```python
from build123d import *

# Parameters (mm, degrees)
SKETCH1_R           = 2.5
BOSS_EXTRUDE1_DEPTH = 45
SKETCH2_R           = 2.5
SKETCH2_R_2         = 2
CUT_EXTRUDE1_DEPTH  = 8
SKETCH3_R           = 2.5
SKETCH3_R_2         = 2
CUT_EXTRUDE2_DEPTH  = 8


with BuildPart() as part:
    # Sketch1 → Boss-Extrude1 (new body, symmetric)
    with BuildSketch(Plane(origin=(0, 0, 0), x_dir=(0, 0, -1), z_dir=(1, 0, 0))):
        Circle(SKETCH1_R)
    extrude(amount=BOSS_EXTRUDE1_DEPTH, both=True)

    # Sketch2 → Cut-Extrude1 (cut)
    with BuildSketch(Plane(origin=(45, 0, 0), x_dir=(0, 0, -1), z_dir=(1, 0, 0))):
        Circle(SKETCH2_R)
        Circle(SKETCH2_R_2, mode=Mode.SUBTRACT)
    extrude(amount=-CUT_EXTRUDE1_DEPTH, mode=Mode.SUBTRACT)

    # Sketch3 → Cut-Extrude2 (cut)
    with BuildSketch(Plane.ZY.offset(45)):
        Circle(SKETCH3_R)
        Circle(SKETCH3_R_2, mode=Mode.SUBTRACT)
    extrude(amount=-CUT_EXTRUDE2_DEPTH, mode=Mode.SUBTRACT)


solid = part.part
```
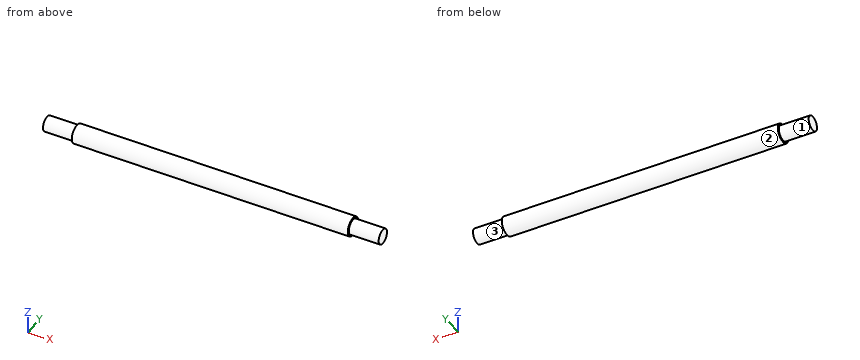
Check sheet for the modelled part. Datum: model origin and axes. Units: mm. Face numbers are marked on the shaded views. A direction names the side the tool comes from. Give positions to 0.01 mm unless a question says otherwise; leave off trailing zeros. Order: outer loops, then holes, each group sorted by start corner. A loop starts at its lowest first (then second) coordinate and runs counter-clockwise, first axis right, second up. Notation, with made-up numbers: (-37.5, -37.75) -> (14.5, -37.75) arc R28 ccw to (14.5, -6.75) -> close; hole circle Ø8 at (54.25, 17). An arc over 180 degrees is marked (long way). Return JSON: item names as keys, results as strings.
1. Material ranges on probe 1 along Z at (x, y) = (19, -1.5); probe 2 along X at (y, z) = (2.1, 0.4); probe 3 along Z at (x, y) = (-28, 0.3), recorded low to high. Write a range as [from, to].
From the geometry:
{"probe 1": "[-2, 2]", "probe 2": "[-37, 37]", "probe 3": "[-2.48, 2.48]"}
2. Go/stop test with a flat-tipped pin: P1, Ø1, axis at x = 24, z = -1, coming from the -Y side. Record where the tip stops, or that it passes through.
From the geometry:
{"P1": "y = -2.45"}
3. Cross-section at C-C, the plane x = -5. Record the cut outline in (y, z), plus the area to 3 significant figures.
From the geometry:
{"outline": "circle Ø5 at (0, 0)", "area": "19.6 mm^2"}
4. Set-up check for the marked faces 1, 2 and 3: record each of +Z, -Z, +X, -X, +Y, -Y from which the full face is reachable in a straight line by a thin tool's end or side.
From the geometry:
{"face 1": "-X", "face 2": "+X, -X", "face 3": "+X"}
5. Cross-section at A-A, the plane z = 0. Record the cut outline in (x, y), plus the area to 3 significant figures.
From the geometry:
{"outline": "(-45, -2) -> (-37, -2) -> (-37, -2.5) -> (37, -2.5) -> (37, -2) -> (45, -2) -> (45, 2) -> (37, 2) -> (37, 2.5) -> (-37, 2.5) -> (-37, 2) -> (-45, 2) -> close", "area": "434 mm^2"}
